Part model, mm, in its own coordinate system. A direction names the side the tool comes from. Round coordinates to 2 decimals unless told otherwise and drop trailing zeros. Write each loop counter-clockwise with the first axis right and the second up, starting at its lowest first coordinate (ties: lowest second). Pieces come first, ordered by that corner, then holes.
from build123d import *

# Parameters (mm, degrees)
F0_W     = 38.1
F0_H     = 38.1
F1_DEPTH = 25.4
F3_DEPTH = 25.4
F5_DEPTH = 25.4


with BuildPart() as f1:
    # F0 (on Front) → F1 (new body)
    with BuildSketch(Plane.XZ):
        with Locations((19.05, 19.05)):
            Rectangle(F0_W, F0_H)
    extrude(amount=F1_DEPTH)

    # F2 (on face) → F3 (cut)
    with BuildSketch(Plane.XZ.offset(25.4)):
        Polygon((0, 0), (12.7, 38.1), (0, 38.1), align=None)
        Polygon((38.1, 38.1), (25.4, 38.1), (38.1, 0), align=None)
    extrude(amount=-F3_DEPTH, mode=Mode.SUBTRACT)

    # F4 (on face) → F5 (cut)
    with BuildSketch(Plane.XZ.offset(25.4)):
        Polygon((12.7, 0), (19.05, 0), (25.4, 0), (25.4, 6.35), (12.7, 6.35), align=None)
    extrude(amount=-F5_DEPTH, mode=Mode.SUBTRACT)


solid = f1.part
Q1. Tool access for faces 1 (the flat face through (19, 0, 15)), 2 (the flat face through (25.4, -13, 3)): list every direction of +Z, -Z, +X, -X, +Y, -Y with a clear straight run to the whole face (end or side of a thin tool).
Q2. Two-plate mould, pull along X, no slides. Class faces 3 (the flat face through (31.66, -12.88, 19.32)), 4 (the flat face through (6.26, -12.88, 18.78)), 5 (the flat face through (19, -25.4, 15)), 6 (the flat face through (12.7, -13, 3)): released by +X, released by -X, zero draft, split by the parting line, or undercut.
Q3. Saw through at D-D, the plane z = 31.5. Write the cut outline in (x, y).
Q4. Saw through at C-C, the plane x = 18. Write the cut outline in (y, z), and give its area (3 significant figures).
Q5. Wall check: line 1 (Z direction, x = 16, y = -13.5); line 2 (X direction, y = -8.25, z = 4.5); line 3 (X direction, y = -0.75, z = 6). Give the ranges that are in metal, low to high.
Q6. Drop flat-ended pins along their axis: P1, Ø12, axis at y = -9, z = 14, coming from the +X side; P2, Ø5, axis at y = -10, z = 4, coming from the +X side; P3, Ø5, axis at y = -20, z = 19, coming from the +X side. Give the stop position or say it passes through.
Q7. Saw through at B-B, the plane y = -21. Write the cut outline in (x, z).
Q8. Saw through at A-A, the plane z = 4.5. Write the cut outline in (x, y).
Computed:
1. face 1: +Z, -Z, +X, -X, +Y
1. face 2: -Z, +Y, -Y
2. face 3: released by +X
2. face 4: released by -X
2. face 5: zero draft
2. face 6: undercut
3. outline: (10.5, -25.4) - (27.6, -25.4) - (27.6, 0) - (10.5, 0) - close
4. outline: (-25.4, 6.35) - (0, 6.35) - (0, 38.1) - (-25.4, 38.1) - close
4. area: 806 mm2
5. line 1: z = 6.35 to 38.1
5. line 2: x = 1.5 to 12.7, 25.4 to 36.6
5. line 3: x = 2 to 12.7, 25.4 to 36.1
6. P1: stops at x = 35.43
6. P2: stops at x = 37.6
6. P3: stops at x = 32.6
7. outline: (0, 0) - (12.7, 0) - (12.7, 6.35) - (25.4, 6.35) - (25.4, 0) - (38.1, 0) - (25.4, 38.1) - (12.7, 38.1) - close
8. outline: (1.5, -25.4) - (12.7, -25.4) - (12.7, 0) - (1.5, 0) - close; (25.4, -25.4) - (36.6, -25.4) - (36.6, 0) - (25.4, 0) - close
